Part model, mm, in its own coordinate system. Round coordinates to 2 decimals unless told otherwise and drop trailing zeros. Write each loop counter-clockwise with the first axis right and the second up, starting at its lowest first coordinate (ties: lowest second). Pieces come first, ordered by that corner, then holes. Notation, with made-up numbers: (74, 57.25) -> (105, 57.25) arc R32 ccw to (105, 93.25) -> close; hole circle Ø8 at (54.5, 28). An arc over 180 degrees is marked (long way). Return JSON: item names as keys, results as strings. Group by question number.
(1) Mould opens along Z. For faces 1 (the flat face through (3, 0, 15)), 2 (the cylindrical face through (13.32, -1.5, -16.77)), 3 (the flat face through (-12.556, -1.503, 62.561)), 4 (the flat face through (13.537, -1.503, 11.167)) say: +Z half, -Z half, draft (parallel to the pull), parting line (faces both ways), or undercut.
(2) Saw through at B-B (z = 7.5). List the corners of the cut face in (x, y), plus the area to 3 significant figures.
(3) Drill centre lines: L1, parallel to Z at x = 44.5, y = -1.7; L2, parallel to X at y = -1.05, z = 37.5; L3, parallel to Z at x = 32.5, y = -0.6. Where is each one in solid material? Low to high. Write a range as from..to.
(4) Saw through at C-C (x = 32). List the corners of the cut face in (y, z).
(5) Drop flat-ended pins along their axis: pin 1 Ø1 at (x, y) = (7, -1) entering from -Z; pin 2 Ø1.5 at (x, y) = (34.5, -1) entering from +Z. Give the stop position or say it passes through.
from build123d import *

# Parameters (mm, degrees)
F0_R     = 1.5875
F1_DEPTH = 3.048


with BuildPart() as f1:
    # F0 (on Front) → F1 (new body)
    with BuildSketch(Plane.XZ):
        with BuildLine():
            Line((-15.100703, 30.326465), (-15.750488, 37.208226))
            ThreePointArc((-15.750488, 37.208226), (-15.804704, 33.731549), (-15.100703, 30.326465))
        make_face()
        with BuildLine():
            ThreePointArc((-9.450293, 87.214476), (-0.596483, 76.517546), (9.525, 86.023851))
            ThreePointArc((9.525, 86.023851), (9.514734, 86.465966), (9.483957, 86.907129))
            ThreePointArc((9.483957, 86.907129), (0.154593, 95.547596), (-9.450293, 87.214476))
        make_face()
        with Locations((0, 86.023851)):
            Circle(F0_R, mode=Mode.SUBTRACT)
        with BuildLine():
            ThreePointArc((9.525, -28.276149), (-0.448187, -18.761699), (-9.482822, -29.17153))
            ThreePointArc((-9.482822, -29.17153), (-6.283976, -35.434171), (0.340179, -37.795073))
            ThreePointArc((0.340179, -37.795073), (6.854408, -34.889977), (9.525, -28.276149))
        make_face()
        with Locations((0, -28.276149)):
            Circle(F0_R, mode=Mode.SUBTRACT)
        with BuildLine():
            ThreePointArc((44.733482, -20.343713), (36.5125, -28.276149), (44.733482, -36.208585))
            ThreePointArc((44.733482, -36.208585), (50.162007, -33.787672), (52.3875, -28.276149))
            ThreePointArc((52.3875, -28.276149), (50.162007, -22.764626), (44.733482, -20.343713))
        make_face()
        with Locations((44.45, -28.276149)):
            Circle(F0_R, mode=Mode.SUBTRACT)
        with BuildLine():
            ThreePointArc((9.483957, 86.907129), (9.514734, 86.465966), (9.525, 86.023851))
            ThreePointArc((9.525, 86.023851), (-0.596483, 76.517546), (-9.450293, 87.214476))
            Line((-9.450293, 87.214476), (-15.750488, 37.208226))
            ThreePointArc((-15.750488, 37.208226), (-0.000795, 51.098851), (15.750289, 37.209804))
            Line((15.750289, 37.209804), (9.483957, 86.907129))
        make_face()
        with Locations((-6.508044, 71.749051)):
            Circle(F0_R, mode=Mode.SUBTRACT)
        with BuildLine():
            ThreePointArc((15.795426, 33.636351), (1.691005, 19.439171), (-15.100703, 30.326465))
            Line((-15.100703, 30.326465), (-9.482822, -29.17153))
            ThreePointArc((-9.482822, -29.17153), (-0.448187, -18.761699), (9.525, -28.276149))
            ThreePointArc((9.525, -28.276149), (6.854408, -34.889977), (0.340179, -37.795073))
            Line((0.340179, -37.795073), (44.733482, -36.208585))
            ThreePointArc((44.733482, -36.208585), (36.5125, -28.276149), (44.733482, -20.343713))
            Line((44.733482, -20.343713), (18.9676, -19.422915))
            ThreePointArc((18.9676, -19.422915), (13.2612, -16.70479), (11.341187, -10.682767))
            Line((11.341187, -10.682767), (15.795426, 33.636351))
        make_face()
        with BuildLine():
            ThreePointArc((15.875, 35.223851), (15.843792, 36.218783), (15.750289, 37.209804))
            ThreePointArc((15.750289, 37.209804), (-0.000795, 51.098851), (-15.750488, 37.208226))
            Line((-15.750488, 37.208226), (-15.100703, 30.326465))
            ThreePointArc((-15.100703, 30.326465), (1.691005, 19.439171), (15.795426, 33.636351))
            ThreePointArc((15.795426, 33.636351), (15.855094, 34.429104), (15.875, 35.223851))
        make_face()
        with Locations((0, 35.223851)):
            Circle(F0_R, mode=Mode.SUBTRACT)
        with Locations((-6.508044, 71.749051)):
            Circle(F0_R)
        with Locations((0, 35.223851)):
            Circle(F0_R)
        with Locations((0, 86.023851)):
            Circle(F0_R)
        with Locations((44.45, -28.276149)):
            Circle(F0_R)
        with Locations((0, -28.276149)):
            Circle(F0_R)
    extrude(amount=F1_DEPTH)


solid = f1.part
Computed values:
{
 "1": {"face 1": "draft", "face 2": "undercut", "face 3": "+Z half", "face 4": "undercut"},
 "2": {"outline": "(-12.95, -3.05) -> (13.17, -3.05) -> (13.17, 0) -> (-12.95, 0) -> close", "area": "79.6 mm2"},
 "3": {"L1": "-36.22..-20.34", "L2": "-15.71..15.71", "L3": "-36.65..-19.91"},
 "4": {"outline": "(-3.05, -36.66) -> (0, -36.66) -> (0, -19.89) -> (-3.05, -19.89) -> close"},
 "5": {"pin 1": "z = -37.57", "pin 2": "z = -19.95"}
}
